Design review of the part built by this model. Coordinates are the model's own, in mm. Face numbers are marked on the shaded views. A direction names the side the tool comes from. Coordinates: 2 decimals unless noted, no trailing zeros. Write each loop counter-clockwise with the first axis right and the second up, starting at its lowest first coordinate (ties: lowest second). Pieces come first, ordered by that corner, then holes.
Q1. The part is to be moulded in two halves that separate along X. For the marked faces 1, 2, 3 and 4, say which applies: released by +X, released by -X, zero draft, split by the parting line, or undercut.
Q2. Take a section at B-B, the plane x = 56. Write out the cut boundary in (y, z), plus the area to 3 significant figures.
Q3. For L1, parallel to Y at x = 30, z = 36; L2, parallel to Z at x = 38.5, y = -34.5; L3, parallel to Y at x = 58.5, z = 7, list the stretches that pass through material, from the lowest coordinate up.
Q4. Take a section at D-D, the plane z = 14.5. Write out the cut boundary in (x, y), plus the area to 3 significant figures.
Q5. For pin 1 Ø1 at (x, y) = (65, -19) entering from -Z; pin 2 Ø3 at (y, z) = (-40.5, 21.5) entering from +X; pin 3 Ø6 at (y, z) = (-38, 8) entering from +X; pin 4 Ø3 at (y, z) = (-5.5, 8.5) entering from +X, all flat-tipped, find the tip position at first contact; note any pin that passes through.
Q6. Take a section at C-C, the plane x = 9. Write out the cut boundary in (y, z), plus the area to 3 significant figures.
Q7. For the marked faces 5, 6 and 7, list the 3-axis set-ups (+Z, -Z, +X, -X, +Y, -Y) from which the entire face can be reached by the end or side of a thin tool; tool diameter is ignored.
Q8. Take a section at A-A, the plane y = -29.5. Write out the cut boundary in (x, z).
from build123d import *

# Parameters (mm, degrees)
F1_DEPTH = 50
F3_DEPTH = 15
F4_R     = 7.6198541316
F5_DEPTH = 295


with BuildPart() as f1:
    # F0 (on Front) → F1 (new body)
    with BuildSketch(Plane.XZ):
        Polygon((0, 32.3076955974), (0, 0), (67.7884593606, 0), (44.5192344487, 32.3076955974), align=None)
    extrude(amount=F1_DEPTH)

    # F2 (on Front) → F3 (join)
    with BuildSketch(Plane.XZ):
        Polygon((0, 47.5000031292), (0, 0), (82.8365385532, 0), (51.2980781496, 47.5000031292), align=None)
    extrude(amount=F3_DEPTH)

    # F4 (on Top) → F5 (cut, symmetric)
    with BuildSketch(Plane.XY):
        with Locations((56.1298057437, -28.2692331821)):
            Circle(F4_R)
    extrude(amount=F5_DEPTH, both=True, mode=Mode.SUBTRACT)


solid = f1.part
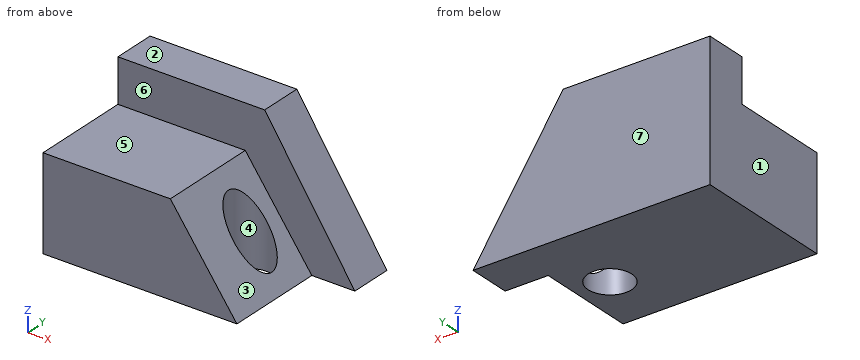
Responses:
1. face 1: released by -X
1. face 2: zero draft
1. face 3: released by +X
1. face 4: undercut
2. outline: (-50, 0) - (-35.89, 0) - (-35.89, 16.37) - (-50, 16.37) - close; (-20.65, 0) - (0, 0) - (0, 40.42) - (-15, 40.42) - (-15, 16.37) - (-20.65, 16.37) - close
2. area: 930 mm2
3. L1: y = -15 to 0
3. L2: z = 0 to 32.31
3. L3: y = -50 to -35.51, -21.03 to 0
4. outline: (0, -50) - (57.35, -50) - (57.35, -35.79) arc R7.62 cw (long way) to (57.35, -20.75) - (57.35, -15) - (73.21, -15) - (73.21, 0) - (0, 0) - close
4. area: 3,000 mm2
5. pin 1: stops at z = 0
5. pin 2: stops at x = 53.38
5. pin 3: stops at x = 64.19
5. pin 4: stops at x = 78.19
6. outline: (-50, 0) - (0, 0) - (0, 47.5) - (-15, 47.5) - (-15, 32.31) - (-50, 32.31) - close
6. area: 1,840 mm2
7. face 5: +Z, +X, -X, -Y
7. face 6: +Z, +X, -Y
7. face 7: +Z, -Z, +X, -X, +Y
8. outline: (0, 0) - (48.61, 0) - (48.61, 26.63) - (44.52, 32.31) - (0, 32.31) - close; (63.65, 0) - (67.79, 0) - (63.65, 5.75) - close
